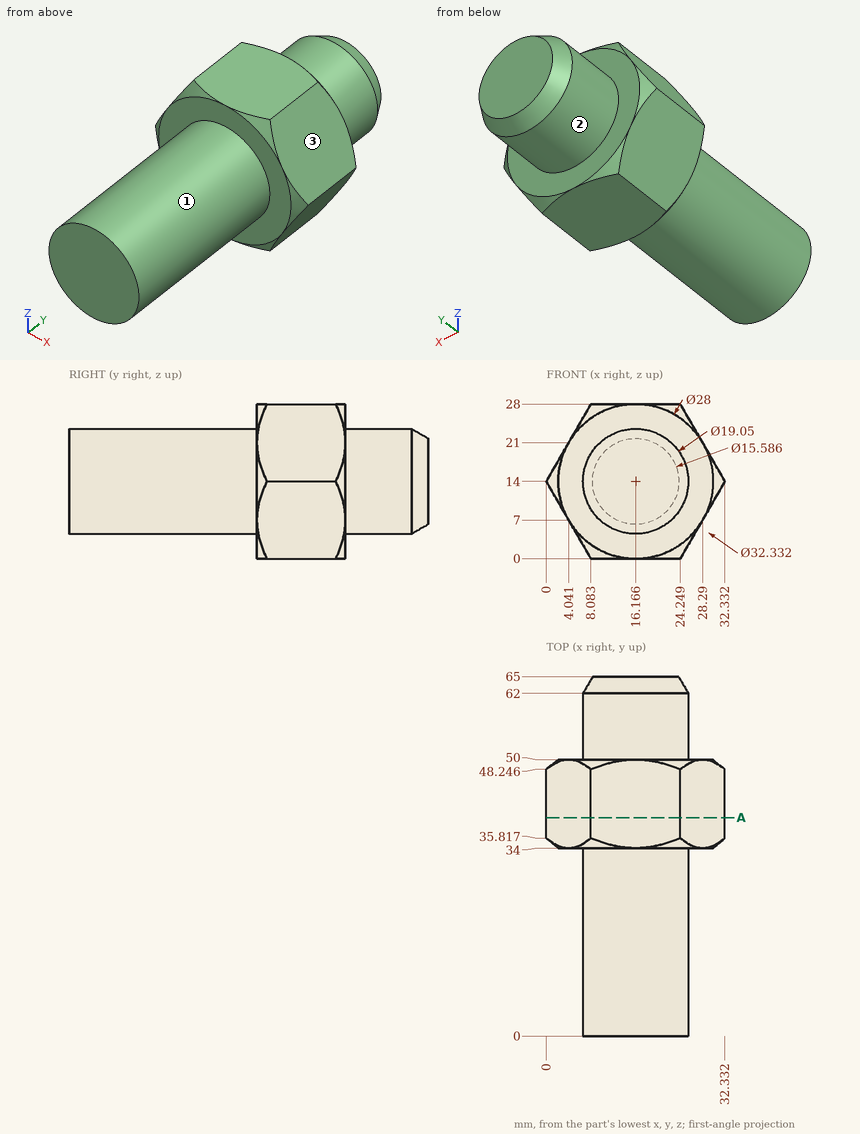
Geometry: see drawing. Coordinates: mm, zero at the bounding-box minimum. A direction names the side the tool comes from. Coordinates: 2 decimals unless noted, no trailing zeros. Order: outer loops, then holes, each group sorted by start corner. A loop starts at its lowest first (then second) coordinate and runs counter-clockwise, first axis right, second up. Notation, with made-up numbers: (89.5, 35.5) - (129.5, 35.5) arc R18 ccw to (129.5, 48.5) - close; hole circle Ø1 at (36.25, 10.25). An arc over 180 degrees is marked (long way). Use one line per item in the form item = value.
1) Pin query (flat end, axial travel): pin 1 (5 mm diameter, centred on x = 5, z = 3.5, fed in from +Y); pin 2 (1.5 mm diameter, centred on x = 15.5, z = 23.5, fed in from +Y); pin 3 (2 mm diameter, centred on y = 16.5, z = 18, fed in from +X). Return the tip coordinate at first contact, or that it passes through.
Solutions:
pin_1 = 50
pin_2 = 63.3
pin_3 = 25.21
2) Ray query, L1, parallel to Y at x = 25.5, z = 8.75; L2, parallel to Y at x = 2, z = 15.25 (1 decimal); L3, parallel to Z at x = 4, y = 46.5 (1 decimal). Return the intervals inside material, ascending.
Solutions:
L1 = 34 to 50
L2 = 34.2 to 49.8
L3 = 7.1 to 20.9
3) Set-up query: the marked faces 1, 2 and 3. Return all of +Z, -Z, +X, -X, +Y, -Y with unobstructed straight access to the full face (end or side cutting, diameter ignored); none if empty.
Solutions:
face_1 = -Y
face_2 = +Y
face_3 = +Z, +X, +Y, -Y
4) Section A-A (y = 39.5). Return loops of the section in (x, z), then the cut area to 3 significant figures.
Solutions:
outline = (0, 14) - (8.08, 0) - (24.25, 0) - (32.33, 14) - (24.25, 28) - (8.08, 28) - close
area = 679 mm^2
